Answer from the drawing. Dimensions are ordinates in mm from the lowest x, y and z of the part. A direction names the side the tool comes from. Give positions to 0.01 mm unless a question says otherwise; leave off trailing zeros. Order: outer loops, then holes, each group sorted by start corner. A loop starts at its lowest first (then second) coordinate and runs counter-clockwise, first axis right, second up. Notation, with made-up numbers: (79.5, -27.5) - (102.5, -27.5) arc R24 cw to (102.5, -13.5) - close; hole circle Ø8 at (0.5, 38). An arc over 180 degrees is marked (long way). Write each question's results on one line, items separated by ' | '.
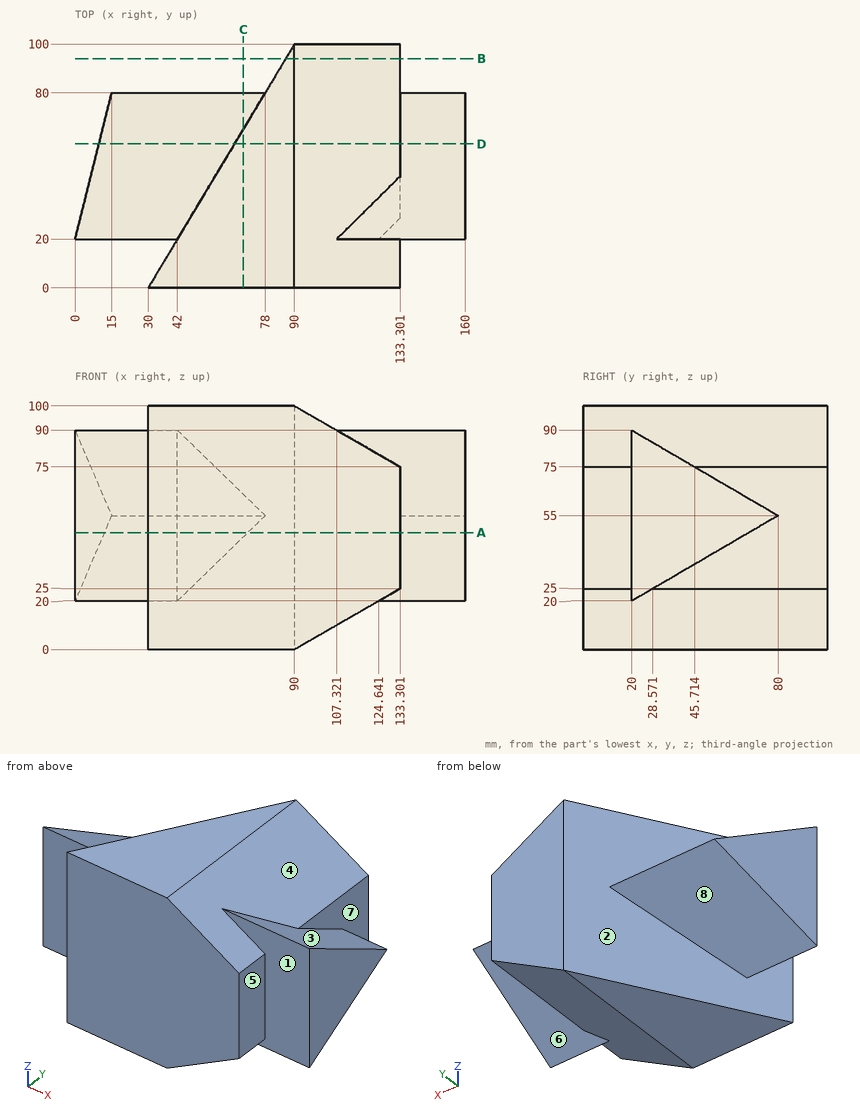
1. Determine the mould class of the marked faces 1, 2, 3 and 4 for opening direction Y: +Y half, -Y half, draft (parallel to the pull), parting line (faces both ways), or undercut.
Answer list:
face 1: -Y half | face 2: undercut | face 3: +Y half | face 4: draft
2. A cutting plane is placed at C-C, the plane x = 69. Write down the section's boundary in (y, z), then the cut area to 3 significant figures.
Answer list:
outline: (0, 0) - (65, 0) - (65, 46.25) - (80, 55) - (65, 63.75) - (65, 100) - (0, 100) - close | area: 6,630 mm^2
3. Straight lines are drawn through the part: line 1 (Y direction, x = 48, z = 21); line 2 (Y direction, x = 13, z = 25) (1 decimal); line 3 (Z direction, x = 114, y = 16.5) (1 decimal). For each, find the intervals that lie inside material, in ascending order. Write a range as [from, to].
Answer list:
line 1: [0, 30] | line 2: [20, 28.6] | line 3: [13.9, 86.1]
4. A cutting plane is placed at D-D, the plane y = 59. Write down the section's boundary in (x, z).
Answer list:
outline: (9.75, 42.75) - (65.4, 42.75) - (65.4, 0) - (90, 0) - (133.3, 25) - (133.3, 42.75) - (160, 42.75) - (160, 67.25) - (133.3, 67.25) - (133.3, 75) - (90, 100) - (65.4, 100) - (65.4, 67.25) - (9.75, 67.25) - close
5. Given P1, Ø2, axis at x = 53.5, z = 75, coming from the +Y side; P2, Ø15, axis at y = 79.5, z = 42, coming from the +X side; P3, Ø5, axis at x = 143, y = 67, coming from the -Z side, each flat-ended and moving along its own axis, determine where each tip first touches the part or whether it passes through.
Answer list:
P1: y = 47.43 | P2: x = 133.3 | P3: z = 45.96
6. A tool of negligible diameter and unlimited length cuts with its end or side. For the marked faces 5, 6, 7 and 8, from which of +Z, -Z, +X, -X, +Y, -Y can it reach the whole face along a straight path? Write none if from no direction.
Answer list:
face 5: +Z, -Z, +X, -Y | face 6: -Z, +X, +Y | face 7: +X, +Y | face 8: -Z, -X, +Y
7. A cutting plane is placed at A-A, the plane z = 48. Write down the section's boundary in (x, y).
Answer list:
outline: (0, 20) - (42, 20) - (30, 0) - (133.3, 0) - (133.3, 20) - (160, 20) - (160, 68) - (133.3, 68) - (133.3, 100) - (90, 100) - (70.8, 68) - (12, 68) - close
8. A cutting plane is placed at B-B, the plane y = 94. Write down the section's boundary in (x, z), then the cut area to 3 significant figures.
Answer list:
outline: (86.4, 0) - (90, 0) - (133.3, 25) - (133.3, 75) - (90, 100) - (86.4, 100) - close | area: 3,610 mm^2
